from build123d import *

# Parameters (mm, degrees)
SKETCH1_R               = 2
SKETCH1_R_2             = 2.075
PRIMARY_DEPTH           = 4
SWINGYBIT_PIN_START     = -4
SKETCH7_R               = 7.5
SKETCH7_R_2             = 2
SWINGYBIT_PIN_EXT_DEPTH = 6
WHEEL_PIN_START         = -4
SKETCH8_R               = 5
SKETCH8_R_2             = 2
SKETCH8_R_3             = 8.75
WHEEL_PIN_EXT_DEPTH     = 1.75
SKETCH10_W              = 42.5
SKETCH10_H              = 12.5
WINDOW_CUT_DEPTH        = 11
FILLET1_R               = 2
CHAMFER1_SIZE           = 0.5
CHAMFER1_SIZE2          = 0.866025404
CHAMFER1_PART_2_SIZE    = 0.5
CHAMFER1_PART_2_SIZE2   = 0.866025404
CHAMFER1_PART_3_SIZE    = 0.5
CHAMFER1_PART_3_SIZE2   = 0.866025404
CHAMFER1_PART_4_SIZE    = 0.5
CHAMFER1_PART_4_SIZE2   = 0.866025404
CHAMFER1_PART_5_SIZE    = 0.5
CHAMFER1_PART_5_SIZE2   = 0.866025404


with BuildPart() as part:
    # Sketch1 → Primary (new body)
    with BuildSketch(Plane(origin=(0, 0, 0), x_dir=(1, 0, 0), z_dir=(0, 1, 0))):
        Polygon((0, 0), (-23, -20), (-23, -90), (44, -90), (44, -82.5), (213, -82.5), (233, -77.5), (233, 0), align=None)
        with Locations((16, -6)):
            Circle(SKETCH1_R, mode=Mode.SUBTRACT)
        with Locations((30, -40.5)):
            Circle(SKETCH1_R_2, mode=Mode.SUBTRACT)
        with Locations((54.5, -59.5)):
            Circle(SKETCH1_R, mode=Mode.SUBTRACT)
        with Locations((44.75, -77.5)):
            Circle(SKETCH1_R, mode=Mode.SUBTRACT)
        with Locations((187, -16)):
            Circle(SKETCH1_R, mode=Mode.SUBTRACT)
    extrude(amount=PRIMARY_DEPTH)

    # Sketch7 → Swingybit_Pin Ext (add)
    with BuildSketch(Plane(origin=(0, 4, 0), x_dir=(1, 0, 0), z_dir=(0, 1, 0)).offset(SWINGYBIT_PIN_START)):
        with Locations((187, -16)):
            Circle(SKETCH7_R)
        with Locations((187, -16)):
            Circle(SKETCH7_R_2, mode=Mode.SUBTRACT)
    extrude(amount=-SWINGYBIT_PIN_EXT_DEPTH)

    # Sketch8 → Wheel_Pin Ext (add)
    with BuildSketch(Plane(origin=(0, 4, 0), x_dir=(1, 0, 0), z_dir=(0, 1, 0)).offset(WHEEL_PIN_START)):
        with Locations((16, -6)):
            Circle(SKETCH8_R)
        with Locations((16, -6)):
            Circle(SKETCH8_R_2, mode=Mode.SUBTRACT)
        with Locations((54.5, -59.5)):
            Circle(SKETCH8_R_3)
        with Locations((54.5, -59.5)):
            Circle(SKETCH8_R_2, mode=Mode.SUBTRACT)
    extrude(amount=-WHEEL_PIN_EXT_DEPTH)

    # Sketch10 → Window Cut (cut, through all)
    with BuildSketch(Plane(origin=(0, 4, 0), x_dir=(1, 0, 0), z_dir=(0, 1, 0))):
        with Locations((127.5, -31)):
            Rectangle(SKETCH10_W, SKETCH10_H)
        with BuildLine():
            Line((97.081439654, -48.031479895), (96.132758806, -54.031479895))
            ThreePointArc((96.132758806, -54.031479895), (98.396768435, -57.417387228), (101.949607057, -55.425542407))
            Line((101.949607057, -55.425542407), (103.044628631, -48.5))
            ThreePointArc((103.044628631, -48.5), (100.279610619, -45.509216914), (97.081439654, -48.031479895))
        make_face()
    extrude(amount=-WINDOW_CUT_DEPTH, mode=Mode.SUBTRACT)

    # Fillet1
    fillet1_edges = [part.edges().sort_by_distance(p)[0] for p in [
        (44, 2, 82.5),
        (0, 2, 0),
        (-23, 2, 20),
        (-23, 2, 90),
        (44, 2, 90),
    ]]
    fillet(fillet1_edges, radius=FILLET1_R)

    # Chamfer1
    chamfer1_edges = [part.edges().sort_by_distance(p)[0] for p in [
        (27.925, 0, 40.5),
    ]]
    chamfer1_side = [part.faces().sort_by_distance(p)[0] for p in [
        (27.925, 2, 40.5),
    ]]
    chamfer(chamfer1_edges, length=CHAMFER1_SIZE, length2=CHAMFER1_SIZE2, reference=chamfer1_side[0])

    # Chamfer1 part 2
    chamfer1_part_2_edges = [part.edges().sort_by_distance(p)[0] for p in [
        (42.75, 0, 77.5),
    ]]
    chamfer1_part_2_side = [part.faces().sort_by_distance(p)[0] for p in [
        (42.75, 2, 77.5),
    ]]
    chamfer(chamfer1_part_2_edges, length=CHAMFER1_PART_2_SIZE, length2=CHAMFER1_PART_2_SIZE2, reference=chamfer1_part_2_side[0])

    # Chamfer1 part 3
    chamfer1_part_3_edges = [part.edges().sort_by_distance(p)[0] for p in [
        (185, -6, 16),
    ]]
    chamfer1_part_3_side = [part.faces().sort_by_distance(p)[0] for p in [
        (179.712132034, -6, 16),
    ]]
    chamfer(chamfer1_part_3_edges, length=CHAMFER1_PART_3_SIZE, length2=CHAMFER1_PART_3_SIZE2, reference=chamfer1_part_3_side[0])

    # Chamfer1 part 4
    chamfer1_part_4_edges = [part.edges().sort_by_distance(p)[0] for p in [
        (14, -1.75, 6),
    ]]
    chamfer1_part_4_side = [part.faces().sort_by_distance(p)[0] for p in [
        (11.141421356, -1.75, 6),
    ]]
    chamfer(chamfer1_part_4_edges, length=CHAMFER1_PART_4_SIZE, length2=CHAMFER1_PART_4_SIZE2, reference=chamfer1_part_4_side[0])

    # Chamfer1 part 5
    chamfer1_part_5_edges = [part.edges().sort_by_distance(p)[0] for p in [
        (52.5, -1.75, 59.5),
    ]]
    chamfer1_part_5_side = [part.faces().sort_by_distance(p)[0] for p in [
        (45.997487373, -1.75, 59.5),
    ]]
    chamfer(chamfer1_part_5_edges, length=CHAMFER1_PART_5_SIZE, length2=CHAMFER1_PART_5_SIZE2, reference=chamfer1_part_5_side[0])


solid = part.part
Design review of the part built by this model. Coordinates are the model's own, in mm. A direction names the side the tool comes from. Coordinates: 2 decimals unless noted, no trailing zeros. Loops run counter-clockwise (first coordinate to the right, second up) from the corner with the lowest first, then second, coordinate; pieces in that order, holes last. Notation, with made-up numbers: (20.25, -15.75) - (31.25, -15.75) arc R12 ccw to (31.25, -10.75) - close; hole circle Ø6 at (48.5, -33). An arc over 180 degrees is marked (long way). Use CSV: the item, a comma, the result in double quotes. Start each with the question number.
1. Clearance check with flat-ended pins moving along their axes: pin 1 (4.5 mm diameter, centred on x = 113.5, y = 1, fed in from +Z); pin 2 (9 mm diameter, centred on x = 56.5, z = 61.5, fed in from -Y); pin 3 (3.5 mm diameter, centred on x = 30, z = 40.5, fed in from +Y); pin 4 (1 mm diameter, centred on y = -3.5, z = 14, fed in from +X). State where each tip first meets the part, or that it passes through.
2. Add section B-B on z = 35. Give the boundary of the cut face in (x, y), plus the area to 3 significant figures.
3. Add section A-A on x = 144.5. Give the boundary of the cut face in (y, z), plus the area to 3 significant figures.
4. Mouldability with a two-part tool opening along X and no side actions: class faces 3 (the flat face through (-11.286, 1.972, 9.814)), 4 (the flat face through (18, -1.75, 8)), 5 (the cylindrical face through (29.73, 2.226, 38.443)) as released by +X, released by -X, zero draft, split by the parting line, or undercut.
5. Add section C-C on y = -3.25. Give the boundary of the cut face in (x, z).
6. To check wall thickness, follow probe 1 along Z at (x, y) = (30, 1.75) (3 decimals); probe 2 along X at (y, z) = (2.85, 59.5); probe 3 along Z at (x, y) = (54.5, 1.1). State the ranges of each line that lie inside material, in increasing order.
7. For faces 1 (the cylindrical face through (59.2, -0.86, 52.12)), 2 (the flat face through (103, 4, 44)), list the 3-axis set-ups (+Z, -Z, +X, -X, +Y, -Y) from which the entire face can be reached by the end or side of a thin tool; tool diameter is ignored.
Resolved:
1,pin 1,"z = 82.5"
1,pin 2,"y = -1.75"
1,pin 3,"through"
1,pin 4,"x = 194.35"
2,outline,"(-23, 0) - (106.25, 0) - (106.25, 4) - (-23, 4) - close; (148.75, 0) - (233, 0) - (233, 4) - (148.75, 4) - close"
2,area,"854 mm2"
3,outline,"(0, 0) - (4, 0) - (4, 24.75) - (0, 24.75) - close; (0, 37.25) - (4, 37.25) - (4, 82.5) - (0, 82.5) - close"
3,area,"280 mm2"
4,face 3,"released by -X"
4,face 4,"zero draft"
4,face 5,"undercut"
5,outline,"circle Ø15 at (187, 16); hole circle Ø4 at (187, 16)"
6,probe 1,"0 to 38.425, 42.575 to 90"
6,probe 2,"-23 to 52.5, 56.5 to 233"
6,probe 3,"0 to 57.5, 61.5 to 82.5"
7,face 1,"-Y"
7,face 2,"+Z, -Z, +X, -X, +Y"
